Design review of the part built by this model. Coordinates are the model's own, in mm. Coordinates: 2 decimals unless noted, no trailing zeros. Write each loop counter-clockwise with the first axis right and the second up, starting at its lowest first coordinate (ties: lowest second). Pieces come first, ordered by that corner, then holes. Notation, with made-up numbers: M 10.5,53 L 30.5,53 A9 ccw 30.5,65 Z; hole C -17.75,80.5 d10. An arc over 180 degrees is marked long. One line per question, with ' | ' between items.
from build123d import *

# Parameters (mm, degrees)
SKETCH1_R                                 = 8
BOSS_EXTRUDE1_DEPTH                       = 2.3368
CSK_FOR_6_FLAT_HEAD_MACHINE_SCREW_2_COUNT = 2
CSK_FOR_6_FLAT_HEAD_MACHINE_SCREW_2_PITCH = 10.440306509
CSK_FOR_6_FLAT_HEAD_MACHINE_SCREW_3_COUNT = 2
CSK_FOR_6_FLAT_HEAD_MACHINE_SCREW_3_PITCH = 30.149626863
CSK_FOR_6_FLAT_HEAD_MACHINE_SCREW_4_COUNT = 2
CSK_FOR_6_FLAT_HEAD_MACHINE_SCREW_4_PITCH = 27.041634566
CSK_FOR_6_FLAT_HEAD_MACHINE_SCREW_5_COUNT = 2
CSK_FOR_6_FLAT_HEAD_MACHINE_SCREW_5_PITCH = 26
CSK_FOR_6_FLAT_HEAD_MACHINE_SCREW_6_COUNT = 2
CSK_FOR_6_FLAT_HEAD_MACHINE_SCREW_6_PITCH = 52
CSK_FOR_6_FLAT_HEAD_MACHINE_SCREW_7_COUNT = 2
CSK_FOR_6_FLAT_HEAD_MACHINE_SCREW_7_PITCH = 50.009999
CSK_FOR_6_FLAT_HEAD_MACHINE_SCREW_8_COUNT = 2
CSK_FOR_6_FLAT_HEAD_MACHINE_SCREW_8_PITCH = 43.304156844
CSK_FOR_6_FLAT_HEAD_MACHINE_SCREW_9_COUNT = 2
CSK_FOR_6_FLAT_HEAD_MACHINE_SCREW_9_PITCH = 57.454329689
FILLET1_R                                 = 6.6


with BuildPart() as part:
    # Sketch1 → Boss-Extrude1 (new body)
    with BuildSketch(Plane(origin=(0, 0, 0), x_dir=(0, 0, -1), z_dir=(1, 0, 0))):
        with BuildLine():
            Line((-15.217158613, 9.614472619), (-32.825001396, -18.254069638))
            ThreePointArc((-32.825001396, -18.254069638), (-33.341875677, -18.878440867), (-34, -19.351590767))
            Line((-34, -19.351590767), (-34, -71))
            Line((-34, -71), (34, -71))
            Line((34, -71), (34, -19.351590767))
            ThreePointArc((34, -19.351590767), (33.341875677, -18.878440867), (32.825001396, -18.254069638))
            Line((32.825001396, -18.254069638), (15.217158613, 9.614472619))
            ThreePointArc((15.217158613, 9.614472619), (0, 18), (-15.217158613, 9.614472619))
        make_face()
        Circle(SKETCH1_R, mode=Mode.SUBTRACT)
    extrude(amount=BOSS_EXTRUDE1_DEPTH)

    # Sketch4 → CSK for _6 Flat Head Machine Screw _100 (revolve, cut)
    with BuildSketch(Plane(origin=(2.3368, -66, 26), x_dir=(0, 0, -1), z_dir=(0, 1, 0))):
        Polygon((0, 0), (0, 2.3368), (1.8288, 2.3368), (1.8288, 1.438636318), (3.5433, 0), align=None)
    csk_for_6_flat_head_machine_screw_100 = revolve(axis=Axis((8.6868, -66, 26), (-1, 0, 0)), mode=Mode.SUBTRACT)

    # CSK for _6 Flat Head Machine Screw _ 2: CSK for _6 Flat Head Machine Screw _100 ×2
    with Locations(*[Vector(0, 0.957826285, -0.287347886) * (i * CSK_FOR_6_FLAT_HEAD_MACHINE_SCREW_2_PITCH) for i in range(1, CSK_FOR_6_FLAT_HEAD_MACHINE_SCREW_2_COUNT)]):
        add(csk_for_6_flat_head_machine_screw_100, mode=Mode.SUBTRACT)

    # CSK for _6 Flat Head Machine Screw _ 3: CSK for _6 Flat Head Machine Screw _100 ×2
    with Locations(*[Vector(0, 0.99503719, -0.099503719) * (i * CSK_FOR_6_FLAT_HEAD_MACHINE_SCREW_3_PITCH) for i in range(1, CSK_FOR_6_FLAT_HEAD_MACHINE_SCREW_3_COUNT)]):
        add(csk_for_6_flat_head_machine_screw_100, mode=Mode.SUBTRACT)

    # CSK for _6 Flat Head Machine Screw _ 4: CSK for _6 Flat Head Machine Screw _100 ×2
    with Locations(*[Vector(0, 0.832050294, -0.554700196) * (i * CSK_FOR_6_FLAT_HEAD_MACHINE_SCREW_4_PITCH) for i in range(1, CSK_FOR_6_FLAT_HEAD_MACHINE_SCREW_4_COUNT)]):
        add(csk_for_6_flat_head_machine_screw_100, mode=Mode.SUBTRACT)

    # CSK for _6 Flat Head Machine Screw _ 5: CSK for _6 Flat Head Machine Screw _100 ×2
    with Locations(*[(0, 0, -i * CSK_FOR_6_FLAT_HEAD_MACHINE_SCREW_5_PITCH) for i in range(1, CSK_FOR_6_FLAT_HEAD_MACHINE_SCREW_5_COUNT)]):
        add(csk_for_6_flat_head_machine_screw_100, mode=Mode.SUBTRACT)

    # CSK for _6 Flat Head Machine Screw _ 6: CSK for _6 Flat Head Machine Screw _100 ×2
    with Locations(*[(0, 0, -i * CSK_FOR_6_FLAT_HEAD_MACHINE_SCREW_6_PITCH) for i in range(1, CSK_FOR_6_FLAT_HEAD_MACHINE_SCREW_6_COUNT)]):
        add(csk_for_6_flat_head_machine_screw_100, mode=Mode.SUBTRACT)

    # CSK for _6 Flat Head Machine Screw _ 7: CSK for _6 Flat Head Machine Screw _100 ×2
    with Locations(*[Vector(0, 0.199960012, -0.979804059) * (i * CSK_FOR_6_FLAT_HEAD_MACHINE_SCREW_7_PITCH) for i in range(1, CSK_FOR_6_FLAT_HEAD_MACHINE_SCREW_7_COUNT)]):
        add(csk_for_6_flat_head_machine_screw_100, mode=Mode.SUBTRACT)

    # CSK for _6 Flat Head Machine Screw _ 8: CSK for _6 Flat Head Machine Screw _100 ×2
    with Locations(*[Vector(0, 0.519580605, -0.854421439) * (i * CSK_FOR_6_FLAT_HEAD_MACHINE_SCREW_8_PITCH) for i in range(1, CSK_FOR_6_FLAT_HEAD_MACHINE_SCREW_8_COUNT)]):
        add(csk_for_6_flat_head_machine_screw_100, mode=Mode.SUBTRACT)

    # CSK for _6 Flat Head Machine Screw _ 9: CSK for _6 Flat Head Machine Screw _100 ×2
    with Locations(*[Vector(0, 0.52215386, -0.852851304) * (i * CSK_FOR_6_FLAT_HEAD_MACHINE_SCREW_9_PITCH) for i in range(1, CSK_FOR_6_FLAT_HEAD_MACHINE_SCREW_9_COUNT)]):
        add(csk_for_6_flat_head_machine_screw_100, mode=Mode.SUBTRACT)

    # Fillet1
    fillet1_edges = [part.edges().sort_by_distance(p)[0] for p in [
        (1.1684, -71, -34),
        (1.1684, -71, 34),
    ]]
    fillet(fillet1_edges, radius=FILLET1_R)


solid = part.part
1. Insertion check: pin 1 Ø3 at (y, z) = (-56, 23) entering from +X; pin 2 Ø1 at (x, z) = (1.5, 11.5) entering from +Y; pin 3 Ø6 at (y, z) = (-56, -23) entering from +X; pin 4 Ø4 at (y, z) = (-66, 26) entering from +X. Each pin has a flat end and moves straight along its axis. Give the tip position at first contact, or say it passes through.
Answer sheet:
pin 1: through | pin 2: y = 14.25 | pin 3: x = 1.88 | pin 4: x = 1.04
2. Draft analysis for pull direction Y (two halves, no side actions). For faces 1 (the face through (1.152, -4.125, 23.898)), 2 (the face through (0.455, -37.236, 24.348)), 3 (the face through (1.185, -69.015, 32.118)), state which applies: pulls with the +Y half, pulls with the -Y half, needs draft (parallel to the pull), parting line crosses it, or undercut.
Answer sheet:
face 1: pulls with the +Y half | face 2: undercut | face 3: pulls with the -Y half
3. Take a section at B-B (y = -36). Write out the cut boundary in (x, z).
Answer sheet:
outline: M 0,-34 L 2.34,-34 L 2.34,-26.54 L 0.9,-24.83 L 0,-24.83 Z; M 0,-21.17 L 0.9,-21.17 L 2.34,-19.46 L 2.34,19.46 L 0.9,21.17 L 0,21.17 Z; M 0,24.83 L 0.9,24.83 L 2.34,26.54 L 2.34,34 L 0,34 Z
4. Take a section at A-A (z = 0). Write out the cut boundary in (x, y).
Answer sheet:
outline: M 0,-71 L 2.34,-71 L 2.34,-69.54 L 0.9,-67.83 L 0,-67.83 Z; M 0,-64.17 L 0.9,-64.17 L 2.34,-62.46 L 2.34,-8 L 0,-8 Z; M 0,8 L 2.34,8 L 2.34,18 L 0,18 Z
5. Take a section at D-D (x = 1.3). Count the separate pieces of the cut face and the enclosed holes in it, then the cut area to 3 significant figures.
Answer sheet:
separate pieces: 1 | enclosed holes: 10 | area: 4,730 mm^2
6. Take a section at C-C (y = -3.5). Write out the cut boundary in (x, z).
Answer sheet:
outline: M 0,-23.5 L 2.34,-23.5 L 2.34,-7.19 L 0,-7.19 Z; M 0,7.19 L 2.34,7.19 L 2.34,23.5 L 0,23.5 Z
7. To check wall thickness, follow line 1 along Y through (x, z) = (0.7, 0); line 2 along Y through (x, z) = (2, -22); line 3 along Z through (x, y) = (0.4, -66). State the ranges of each line that lie inside material, in increasing order. Write a range as [from, to].
Answer sheet:
line 1: [-71, -67.83], [-64.17, -8], [8, 18] | line 2: [-71, -58.98], [-53.02, -38.98], [-33.02, -1.12] | line 3: [-33.8, -27.83], [-24.17, -1.83], [1.83, 24.17], [27.83, 33.8]
